Here's how the part is built. I have some questions about the finished solid (model axes, mm). Face numbers are marked on the shaded views. A direction names the side the tool comes from. Round coordinates to 2 decimals unless told otherwise and drop trailing zeros. Write each loop counter-clockwise with the first axis right and the second up, starting at its lowest first coordinate (ties: lowest second). Pieces come first, ordered by that corner, then holes. Notation, with made-up numbers: M -6.75,-20 L 11.25,-20 A26 ccw 11.25,19 Z; hole C 67,-32 d2. An arc over 180 degrees is marked long. Use a Markdown table: item, result. Add a question column.
```python
from build123d import *

# Parameters (mm, degrees)
SKETCH1_R           = 12.7
SKETCH1_R_2         = 8.2
SKETCH1_R_3         = 6.7
BOSS_EXTRUDE1_DEPTH = 20
BOSS_EXTRUDE2_START = 20
SKETCH1_4_R         = 8.2
SKETCH1_4_R_2       = 6.7
BOSS_EXTRUDE2_DEPTH = 20
CHAMFER1_SIZE       = 10
CHAMFER1_SIZE2      = 2.679491924


with BuildPart() as part:
    # Sketch1 → Boss-Extrude1 (new body)
    # profile 1 of 2: a face of its own
    with BuildSketch(Plane.XY):
        Circle(SKETCH1_R)
        Circle(SKETCH1_R_2, mode=Mode.SUBTRACT)
    # profile 2 of 2: a face of its own
    with BuildSketch(Plane.XY):
        Circle(SKETCH1_R_2)
        Circle(SKETCH1_R_3, mode=Mode.SUBTRACT)
    extrude(amount=BOSS_EXTRUDE1_DEPTH)

    # Sketch1<4> → Boss-Extrude2 (add)
    with BuildSketch(Plane.XY.offset(BOSS_EXTRUDE2_START)):
        Circle(SKETCH1_4_R)
        Circle(SKETCH1_4_R_2, mode=Mode.SUBTRACT)
    extrude(amount=BOSS_EXTRUDE2_DEPTH)

    # Chamfer1
    chamfer1_edges = [part.edges().sort_by_distance(p)[0] for p in [
        (-12.7, 0, 0),
    ]]
    chamfer1_side = [part.faces().sort_by_distance(p)[0] for p in [
        (-12.7, 0, 10),
    ]]
    chamfer(chamfer1_edges, length=CHAMFER1_SIZE, length2=CHAMFER1_SIZE2, reference=chamfer1_side[0])


solid = part.part
```
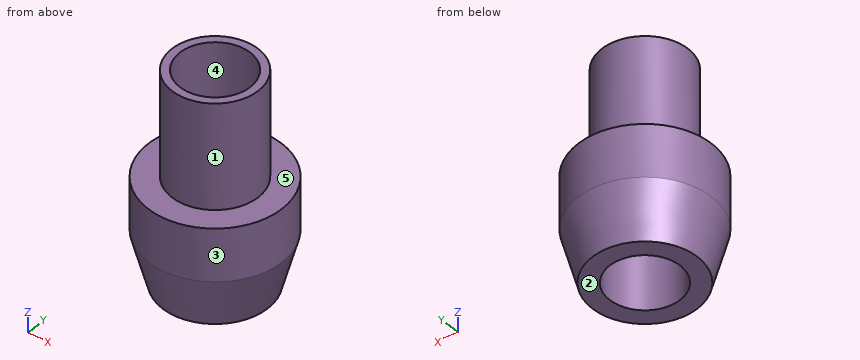
Item 1: Imagine slicing it at A-A on x = 0. List the corners of the cut face in (y, z) for me, plus the area to 3 significant figures.
Item 2: Imagine slicing it at C-C on z = 22.5. List the corners of the cut face in (x, y) for me, plus the area to 3 significant figures.
Item 3: I need wall thicknesses on probe 1 along Y at (x, z) = (0, 19); probe 2 along Y at (x, z) = (0, 20.5); probe 3 along X at (y, z) = (-3, 6). Which ranges of each line are inside material? Lowest first, please. Write a range as from..to.
Item 4: If we mould it in two halves opening along X, with no side actions, what happens to the marked faces 3, 4 and 5? For each: +X half, -X half, draft (parallel to the pull), parting line (faces both ways), or undercut.
Item 5: For pin 1 Ø2 at (x, z) = (4, 10.5) entering from -Y; pin 2 Ø7.5 at (x, y) = (2.5, 0.5) entering from +Z; pin 3 Ø10 at (y, z) = (-6, 18) entering from -X; pin 4 Ø3 at (x, z) = (3, 4.5) entering from +Y, each with a flat end and sliding along its axis, tell me the tip position at first contact or that it passes through.
Item 6: Imagine slicing it at D-D on z = 14. List the corners of the cut face in (x, y) for me.
Item 7: On a 3-axis mill with a long thin cutter (end or side, diameter ignored), from which of +Z, -Z, +X, -X, +Y, -Y can I reach the whole of each face in a straight line? I mean the marked faces 1 and 2. Say none if no direction works.
The answers:
| question | item | result |
|---|---|---|
| 1 | outline | M -12.7,10 L -10.02,0 L -6.7,0 L -6.7,40 L -8.2,40 L -8.2,20 L -12.7,20 Z; M 6.7,0 L 10.02,0 L 12.7,10 L 12.7,20 L 8.2,20 L 8.2,40 L 6.7,40 Z |
| 1 | area | 273 mm² |
| 2 | outline | C 0,0 d16.4; hole C 0,0 d13.4 |
| 2 | area | 70.2 mm² |
| 3 | probe 1 | -12.7..-6.7, 6.7..12.7 |
| 3 | probe 2 | -8.2..-6.7, 6.7..8.2 |
| 3 | probe 3 | -11.23..-5.99, 5.99..11.23 |
| 4 | face 3 | parting line |
| 4 | face 4 | undercut |
| 4 | face 5 | draft |
| 5 | pin 1 | y = -12.34 |
| 5 | pin 2 | through |
| 5 | pin 3 | x = -12.66 |
| 5 | pin 4 | y = 11.36 |
| 6 | outline | C 0,0 d25.4; hole C 0,0 d13.4 |
| 7 | face 1 | +Z |
| 7 | face 2 | -Z, +X, -X, +Y, -Y |
